For this review, take the finished solid that the model builds, in its own axes (mm). A direction names the side the tool comes from. Give positions to 0.01 mm unless a question says otherwise; leave off trailing zeros. Order: outer loops, then holes, each group sorted by start corner. A loop starts at its lowest first (then second) coordinate and runs counter-clockwise, first axis right, second up. Notation, with made-up numbers: (-36.5, 71.5) - (12.5, 71.5) arc R18 ccw to (12.5, 102.5) - close; hole circle Ø10 at (37.5, 69). An arc over 180 degrees is marked (long way). Answer as a JSON object with one key per item and string values. Group by question number.
from build123d import *

# Parameters (mm, degrees)
SKETCH_1_W      = 34
SKETCH_1_H      = 34
SKETCH_1_R      = 2
EXTRUDE_1_DEPTH = 4
FILLET_1_R      = 5
SKETCH_2_R      = 6
EXTRUDE_2_DEPTH = 66
CHAMFER_1_SIZE  = 5
CHAMFER_1_SIZE2 = 18.660254038
CHAMFER_2_SIZE  = 2


with BuildPart() as part:
    # Эскиз1 → Бобышка-Вытянуть1 (new body)
    with BuildSketch(Plane(origin=(0, 0, 0), x_dir=(1, 0, 0), z_dir=(0, 1, 0))):
        Rectangle(SKETCH_1_W, SKETCH_1_H)
        with Locations(Location((-12, 12, 0), (0, 0, 270))):
            Circle(SKETCH_1_R, mode=Mode.SUBTRACT)
        with Locations(Location((12, 12, 0), (0, 0, 270))):
            Circle(SKETCH_1_R, mode=Mode.SUBTRACT)
        with Locations(Location((12, -12, 0), (0, 0, 270))):
            Circle(SKETCH_1_R, mode=Mode.SUBTRACT)
        with Locations(Location((-12, -12, 0), (0, 0, 270))):
            Circle(SKETCH_1_R, mode=Mode.SUBTRACT)
    extrude(amount=EXTRUDE_1_DEPTH)

    # Скругление1
    fillet_1_edges = [part.edges().sort_by_distance(p)[0] for p in [
        (17, 2, 17),
        (-17, 2, 17),
        (-17, 2, -17),
        (17, 2, -17),
    ]]
    fillet(fillet_1_edges, radius=FILLET_1_R)

    # Эскиз2 → Бобышка-Вытянуть2 (add)
    with BuildSketch(Plane(origin=(0, 4, 0), x_dir=(1, 0, 0), z_dir=(0, 1, 0))):
        with Locations(Location((0, 0, 0), (0, 0, 270))):
            Circle(SKETCH_2_R)
    extrude(amount=EXTRUDE_2_DEPTH)

    # Эскиз7 → Вырез-Повернуть3 (revolve, cut)
    with BuildSketch(Plane.XY):
        with BuildLine():
            Line((5.5, 70), (0, 70))
            Line((0, 70), (0, 68))
            ThreePointArc((0, 68), (2.979435889, 68.369051304), (5.5, 70))
        make_face()
    revolve(axis=Axis((0, 82.404747685, 0), (0, -1, 0)), mode=Mode.SUBTRACT)

    # Фаска1
    chamfer_1_edges = [part.edges().sort_by_distance(p)[0] for p in [
        (0, 4, -6),
    ]]
    chamfer_1_side = [part.faces().sort_by_distance(p)[0] for p in [
        (0, 4, 16.519167389),
    ]]
    chamfer(chamfer_1_edges, length=CHAMFER_1_SIZE, length2=CHAMFER_1_SIZE2, reference=chamfer_1_side[0])

    # Фаска2
    chamfer_2_edges = [part.edges().sort_by_distance(p)[0] for p in [
        (-12, 4, -14),
        (12, 4, -14),
        (12, 4, 10),
        (-12, 4, 10),
    ]]
    chamfer(chamfer_2_edges, length=CHAMFER_2_SIZE)


solid = part.part
1) For faces 1 (the face through (0, 0, 0)), 2 (the face through (-8, 4, -8)), list the 3-axis set-ups (+Z, -Z, +X, -X, +Y, -Y) from which the entire face can be reached by the end or side of a thin tool; tool diameter is ignored.
2) Consider section B-B (y = 60). Give the boundary of the cut face in (x, z), plus the area to 3 significant figures.
3) Consider section A-A (x = -13). Give the number of separate pieces and of enclosed holes in the cut face, plus the area to 3 significant figures.
4) For line 1 (X direction, y = 1.25, z = 12); line 2 (Y direction, x = 11, z = 7.5); line 3 (Z direction, x = 2.5, y = 65.5), list the stretches that pass through material, from the lowest coordinate up.
5) For pin 1 (3 mm diameter, centred on x = -12, z = 12, fed in from -Y); pin 2 (3 mm diameter, centred on y = 45, z = -2, fed in from +X); pin 3 (6 mm diameter, centred on x = 2, y = 39, fed in from -Z); pin 4 (10 mm diameter, centred on x = 8.5, y = 36, fed in from -Z), all flat-tipped, find the tip position at first contact; note any pin that passes through.
6) Mouldability with a two-part tool opening along X and no side actions: class faces 3 (the face through (14, 1, -12)), 4 (the face through (1.802, 45.999, 5.723)), 5 (the face through (15, 2, 16)) as released by +X, released by -X, zero draft, split by the parting line, or undercut.
Result set:
{
 "1": {"face 1": "+Z, -Z, +X, -X, -Y", "face 2": "+Y"},
 "2": {"outline": "circle Ø12 at (0, 0)", "area": "113 mm2"},
 "3": {"separate pieces": "3", "enclosed holes": "0", "area": "98.8 mm2"},
 "4": {"line 1": "x = -17 to -14, -10 to 10, 14 to 17", "line 2": "y = 0 to 4", "line 3": "z = -5.45 to 5.45"},
 "5": {"pin 1": "passes through", "pin 2": "stops at x = 5.98", "pin 3": "stops at z = -6", "pin 4": "stops at z = -4.87"},
 "6": {"face 3": "undercut", "face 4": "split by the parting line", "face 5": "released by +X"}
}
